CAD build for the part. Positions are in the model's coordinates, mm. Coordinates: 2 decimals unless noted, no trailing zeros. Order: outer loops, then holes, each group sorted by start corner. A loop starts at its lowest first (then second) coordinate and runs counter-clockwise, first axis right, second up. Notation, with made-up numbers: (34, -18) - (76, -18) arc R25 cw to (76, 20) - close; hole circle Ø9 at (86, -14.5). An arc over 180 degrees is marked (long way). Use one line per item in the form item = value.
```python
from build123d import *

# Parameters (mm, degrees)
F1_DEPTH = 2.38125
F2_R     = 2.38125
F3_DEPTH = 25.4
F5_DEPTH = 25.4


with BuildPart() as f1:
    # F0 (on Front) → F1 (new body)
    with BuildSketch(Plane.XZ):
        with BuildLine():
            Line((60.325, 19.05), (7.9502, 19.05))
            ThreePointArc((7.9502, 19.05), (2.32856, 16.72144), (0, 11.0998))
            Line((0, 11.0998), (0, 0))
            Line((0, 0), (9.525, 0))
            Line((9.525, 0), (12.110345, 7.626242))
            ThreePointArc((12.110345, 7.626242), (13.473756, 9.517878), (15.663421, 10.319465))
            Line((15.663421, 10.319465), (60.325, 12.7))
            Line((60.325, 12.7), (60.325, 19.05))
        make_face()
    extrude(amount=F1_DEPTH)

    # F2 (on face) → F3 (cut)
    with BuildSketch(Plane.XZ.offset(2.38125)):
        with Locations((7.9502, 11.0998)):
            Circle(F2_R)
    extrude(amount=-F3_DEPTH, mode=Mode.SUBTRACT)

    # F4 (on face) → F5 (cut)
    with BuildSketch(Plane.XY.offset(19.05)):
        Polygon((60.325, 0), (45.2374, 0), (60.325, -0.79375), align=None)
        Polygon((60.325, -2.38125), (60.325, -1.5875), (45.2374, -2.38125), align=None)
    extrude(amount=-F5_DEPTH, mode=Mode.SUBTRACT)


solid = f1.part
```
Item 1: Drill centre lines: line 1 (X direction, y = -2.1, z = 10); line 2 (Z direction, x = 6, y = -2.1); line 3 (Z direction, x = 14.5, y = -1.6). Where is each one in solid material? Low to high. Write a range as [from, to].
Derived:
line_1 = [0, 5.84], [10.06, 14.3]
line_2 = [0, 9.73], [12.47, 18.81]
line_3 = [10.08, 19.05]
Item 2: Drop a flat-ended pin along its axis: pin 1 (8 mm diameter, centred on x = 49.5, z = 8.5, fed in from -Y). Give the stop position or say it passes through.
Derived:
pin_1 = -2.26
Item 3: Cut at D-D, the plane x = 5. Write the cut outline in (y, z), plus the area to 3 significant figures.
Derived:
outline = (-2.38, 0) - (0, 0) - (0, 18.48) - (-2.38, 18.48) - close
area = 44.0 mm²
Item 4: Cut at B-B, the plane z = 14.75. Write the cut outline in (x, y) (1 decimal).
Derived:
outline = (0.9, -2.4) - (45.2, -2.4) - (60.3, -1.6) - (60.3, -0.8) - (45.2, 0) - (0.9, 0) - close
Item 5: Cut at C-C, the plane x = 18.5. Write the cut outline in (y, z).
Derived:
outline = (-2.38, 10.47) - (0, 10.47) - (0, 19.05) - (-2.38, 19.05) - close
Item 6: Two-plate mould, pull along X, no slides. Class faces 1 (the face through (0, -1, 6)), 2 (the face through (35, -1, 19.05)), 3 (the face through (10.15, -1.21, 10.19)), 4 (the face through (37.682, -1.174, 11.493)): +X half, -X half, draft (parallel to the pull), parting line (faces both ways), or undercut.
Derived:
face_1 = -X half
face_2 = draft
face_3 = undercut
face_4 = +X half
